The listing builds one solid part. Answer for the finished solid, in the listing's coordinates (mm). Round coordinates to 2 decimals unless told otherwise and drop trailing zeros. Write each loop counter-clockwise with the first axis right and the second up, starting at its lowest first coordinate (ties: lowest second). Pieces come first, ordered by that corner, then holes.
Autodesk Inventor part; units mm, degrees
ref_plane "YZ Plane" through (0, 0, 0) normal (1, 0, 0) x (0, 1, 0)
ref_plane "XZ Plane" through (0, 0, 0) normal (0, 1, 0) x (-1, 0, 0)
ref_plane "XY Plane" through (0, 0, 0) normal (0, 0, 1) x (1, 0, 0)
sketch "スケッチ1" plane through (0, 0, 0) normal (1, 0, 0) x (0, 1, 0)
  line L0 (0, 150) -> (0, -150)
  line L1 (-181.5936, 0) -> (756.1348, 0)
  arc A0 (0, 150) -> (0, -150) centre (622.1736, 0) ccw
  arc A1 (0, 150) -> (0, -150) centre (212.3676, 0) ccw
  point P0 (0, 0)
  point P1 (0, 0)
  dimension "d0" = 300
  dimension "d1" = 640
  dimension "d2" = 260
extrude "押し出し1" add sketch "スケッチ1" along normal mid plane 950 contours A0 L1 A1 | A0 A1 L1
fillet "フィレット1" radius 5 1 edges at (0, 0, 150)
fillet "フィレット2" radius 2 1 edges at (0, 0, -150)
sketch "スケッチ2" plane through (475, 0, 0) normal (1, 0, 0) x (0, 0, -1)
  line L0 (-44.0145, -43.8798) -> (-34.1281, -45.3828)
  line L1 (59.0473, -40.8387) -> (49.2667, -42.922)
  arc A0 (-125.4594, -15.3602) -> (141.0102, -6.0726) centre (0, 212.3676) ccw
  point P0 (0, 0)
  dimension "d7" = 10
  dimension "d8" = 10
extrude "押し出し2" cut sketch "スケッチ2" against normal through all
properties part number "element_1" material "CFRP"
1. For a pull along Z with two mould halves and no side action, classify faces 1 (the face through (-6.65, -17.736, -10.73)), 2 (the face through (-6.7, -47.5, -8.3)), 3 (the face through (-6.65, -33.22, 85.36)), 4 (the face through (-6.65, -26.745, -102.104)) as released by +Z, released by -Z, zero draft, split by the parting line, or undercut.
Geometry says:
face 1: undercut
face 2: split by the parting line
face 3: released by +Z
face 4: released by -Z
2. Section A-A on z = 26 is taken. Determine the outline of the cut face in (x, y).
Geometry says:
outline: (-475, -46.33) - (475, -46.33) - (475, -17.3) - (-475, -17.3) - close
3. Given pin 1 (1.5 mm diameter, centred on x = 329, z = -53.5, fed in from -Y); pin 2 (12 mm diameter, centred on x = -19.5, y = -15.5, fed in from +Z); pin 3 (4 mm diameter, centred on x = 372.5, z = 66, fed in from -Y), each flat-ended and moving along its own axis, determine where each tip first touches the part or whether it passes through.
Geometry says:
pin 1: stops at y = -42.18
pin 2: stops at z = 128.05
pin 3: stops at y = -39.63
4. Section B-B on y = -32.5 is taken. Determine the outline of the cut face in (x, z).
Geometry says:
outline: (-475, -87.41) - (475, -87.41) - (475, 87.41) - (-475, 87.41) - close
5. Straight lines are drawn through the part: line 1 along Y through (x, z) = (-430.5, -55); line 2 along Y through (x, z) = (-372, 41); line 3 along Z through (x, y) = (-84, -23.5). For each, find the intervals that lie inside material, in ascending order.
Geometry says:
line 1: y = -41.7 to -15.46
line 2: y = -44.34 to -16.51
line 3: z = -109.39 to 109.39
